Geometry: final body of the model. Coordinates: model frame, mm. Face numbers are marked on the shaded views. A direction names the side the tool comes from. Coordinates: 2 decimals unless noted, no trailing zeros. Order: outer loops, then holes, each group sorted by start corner. A loop starts at its lowest first (then second) coordinate and runs counter-clockwise, first axis right, second up. Notation, with made-up numbers: M 33,-11 L 48,-11 A20 cw 48,1 Z; hole C 1.5,52 d8. An arc over 180 degrees is marked long. One line per question, with ' | ' between items.
from build123d import *

# Parameters (mm, degrees)
F0_W     = 130
F0_H     = 140
F0_R     = 2.5
F1_DEPTH = 8
F2_W     = 130
F2_H     = 15
F3_DEPTH = 60
F4_R     = 21.5
F5_DEPTH = 25


with BuildPart() as f1:
    # F0 (on Front) → F1 (new body)
    with BuildSketch(Plane.XZ):
        Rectangle(F0_W, F0_H)
        with Locations((-50, -46)):
            Circle(F0_R, mode=Mode.SUBTRACT)
        with Locations((-20, -46)):
            Circle(F0_R, mode=Mode.SUBTRACT)
        with Locations((-50, -14)):
            Circle(F0_R, mode=Mode.SUBTRACT)
        with Locations((-20, -14)):
            Circle(F0_R, mode=Mode.SUBTRACT)
        with Locations((20, -46)):
            Circle(F0_R, mode=Mode.SUBTRACT)
        with Locations((50, -46)):
            Circle(F0_R, mode=Mode.SUBTRACT)
        with Locations((20, -14)):
            Circle(F0_R, mode=Mode.SUBTRACT)
        with Locations((50, -14)):
            Circle(F0_R, mode=Mode.SUBTRACT)
        with Locations((-50, 14)):
            Circle(F0_R, mode=Mode.SUBTRACT)
        with Locations((-20, 14)):
            Circle(F0_R, mode=Mode.SUBTRACT)
        with Locations((-50, 46)):
            Circle(F0_R, mode=Mode.SUBTRACT)
        with Locations((-20, 46)):
            Circle(F0_R, mode=Mode.SUBTRACT)
        with Locations((20, 14)):
            Circle(F0_R, mode=Mode.SUBTRACT)
        with Locations((50, 14)):
            Circle(F0_R, mode=Mode.SUBTRACT)
        with Locations((20, 46)):
            Circle(F0_R, mode=Mode.SUBTRACT)
        with Locations((50, 46)):
            Circle(F0_R, mode=Mode.SUBTRACT)
    extrude(amount=F1_DEPTH)

    # F2 (on face) → F3 (join)
    with BuildSketch(Plane.XZ.offset(8)):
        with Locations((0, -62.5)):
            Rectangle(F2_W, F2_H)
    extrude(amount=F3_DEPTH)

    # F4 (on face) → F5 (cut)
    with BuildSketch(Plane.XY.offset(-55)):
        with Locations((0, -41.5)):
            Circle(F4_R)
    extrude(amount=-F5_DEPTH, mode=Mode.SUBTRACT)


solid = f1.part
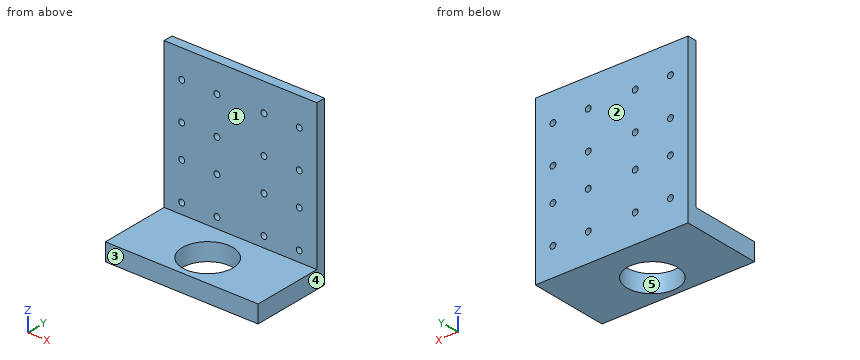
1. Section D-D, the plane x = 0. Output: boundary loops of the cut face in (y, z).
Response values:
outline: M -68,-70 L -63,-70 L -63,-55 L -68,-55 Z; M -20,-70 L 0,-70 L 0,70 L -8,70 L -8,-55 L -20,-55 Z
2. Section A-A, the plane x = 50. Output: boundary loops of the cut face in (y, z).
Response values:
outline: M -68,-70 L 0,-70 L 0,-48.5 L -8,-48.5 L -8,-55 L -68,-55 Z; M -8,-43.5 L 0,-43.5 L 0,-16.5 L -8,-16.5 Z; M -8,-11.5 L 0,-11.5 L 0,11.5 L -8,11.5 Z; M -8,16.5 L 0,16.5 L 0,43.5 L -8,43.5 Z; M -8,48.5 L 0,48.5 L 0,70 L -8,70 Z
3. Pin query (flat end, axial travel): P1, Ø8, axis at x = -50, z = 46, coming from the -Y side; P2, Ø1.5, axis at x = -23.5, y = -57, coming from the +Z side. Return the tip coordinate at first contact, or that it passes through.
Response values:
P1: stops at y = -8 | P2: stops at z = -55
4. Draft query along X for the marked faces 3, 4 and 5. Return one class per face: pulls with the +X half, pulls with the -X half, needs draft (parallel to the pull), parting line crosses it, or undercut.
Response values:
face 3: needs draft | face 4: pulls with the +X half | face 5: undercut
5. Section B-B, the plane z = -57. Output: boundary loops of the cut face in (x, y).
Response values:
outline: M -65,-68 L 65,-68 L 65,0 L -65,0 Z; hole C 0,-41.5 d43
6. Section C-C, the plane y = -34. Output: boundary loops of the cut face in (x, z), and give its area (3 significant figures).
Response values:
outline: M -65,-70 L -20.15,-70 L -20.15,-55 L -65,-55 Z; M 20.15,-70 L 65,-70 L 65,-55 L 20.15,-55 Z | area: 1,350 mm^2
7. Material intervals for line 1 (Z direction, x = -20, y = -3.75); line 2 (Y direction, x = 42.5, z = 16); line 3 (Z direction, x = 49, y = -59.5), sorted ascending. Write a range as [from, to].
Response values:
line 1: z = [-70, -48.5], [-43.5, -16.5], [-11.5, 11.5], [16.5, 43.5], [48.5, 70] | line 2: y = [-8, 0] | line 3: z = [-70, -55]
8. Access query for the marked faces 1 and 2. Directions: +Z, -Z, +X, -X, +Y, -Y. A direction counts if a zero-diameter tool reaches every point of the face in a straight line with its end or side. Return the directions, or none.
Response values:
face 1: +Z, +X, -X, -Y | face 2: +Z, -Z, +X, -X, +Y
